Check sheet for the modelled part. Datum: model origin and axes. Units: mm. A direction names the side the tool comes from. Coordinates: 2 decimals unless noted, no trailing zeros. Order: outer loops, then holes, each group sorted by start corner. A loop starts at its lowest first (then second) coordinate and runs counter-clockwise, first axis right, second up. Notation, with made-up numbers: (85.5, 45) -> (98.5, 45) arc R20 ccw to (98.5, 52) -> close; hole circle Ø4 at (-27, 37). An arc over 180 degrees is marked (long way). Put each result on its own line as item: value. Start each with the question number.
```python
from build123d import *

# Parameters (mm, degrees)
BOSS_EXTRUDE1_DEPTH = 210
FILLET1_R           = 3
FILLET2_R           = 8
SKETCH2_R           = 3.5
SKETCH2_R_2         = 1.6
SKETCH2_W           = 10
SKETCH2_H           = 25
CUT_EXTRUDE1_DEPTH  = 111
CHAMFER1_SIZE       = 30


with BuildPart() as part:
    # Sketch1 → Boss-Extrude1 (new body)
    with BuildSketch(Plane(origin=(0, 0, 0), x_dir=(0, 0, -1), z_dir=(1, 0, 0))):
        Polygon((0, 190), (0, 0), (-110, 0), (-110, 5), (-5, 5), (-5, 190), align=None)
    extrude(amount=BOSS_EXTRUDE1_DEPTH)

    # Fillet1
    fillet1_edges = [part.edges().sort_by_distance(p)[0] for p in [
        (105, 5, 5),
    ]]
    fillet(fillet1_edges, radius=FILLET1_R)

    # Fillet2
    fillet2_edges = [part.edges().sort_by_distance(p)[0] for p in [
        (105, 0, 0),
    ]]
    fillet(fillet2_edges, radius=FILLET2_R)

    # Sketch2 → Cut-Extrude1 (cut, through all)
    with BuildSketch(Plane(origin=(0, 0, 0), x_dir=(-1, 0, 0), z_dir=(0, 0, -1))):
        with Locations((-105, 120)):
            Circle(SKETCH2_R)
        with Locations((-105, 15)):
            Circle(SKETCH2_R_2)
        with Locations((-105, 32.5)):
            Rectangle(SKETCH2_W, SKETCH2_H)
    extrude(amount=-CUT_EXTRUDE1_DEPTH, mode=Mode.SUBTRACT)

    # Chamfer1
    chamfer1_edges = [part.edges().sort_by_distance(p)[0] for p in [
        (210, 190, 2.5),
        (0, 190, 2.5),
    ]]
    chamfer(chamfer1_edges, length=CHAMFER1_SIZE)


solid = part.part
```
1) Gauge pin test, flat ends, axial feed: pin 1 (3.5 mm diameter, centred on x = 105, y = 15, fed in from +Z); pin 2 (3 mm diameter, centred on x = 93.5, z = 93.5, fed in from +Y); pin 3 (1.5 mm diameter, centred on x = 107, z = 1.5, fed in from -Y). Record the tip position at first contact, or that the pin passes through.
2) Scan lines: line 1 along Y through (x, z) = (105, 2.7); line 2 along Y through (x, z) = (105, 3.8); line 3 along Y through (x, z) = (117.5, 84.5). Record each from-to range of solid material in increasing order. Write a range as [from, to].
3) Sectioned sample at D-D (z = 54). Record the boundary of the cut face in (x, y).
4) Sectioned sample at A-A (y = 120). Record the boundary of the cut face in (x, z), plus the area to 4 significant figures.
5) Mould release check, pull along X, two halves, no side actions. Record for faces 4 (the flat face through (0, 45, 2)), 5 (the flat face through (104, 190, 3)), 6 (the flat face through (105, 20, 2)): +X half, -X half, draft (parallel to the pull), parting line (faces both ways), or undercut.
6) Sectioned sample at B-B (x = 149). Record the boundary of the cut face in (y, z), plus the area to 3 significant figures.
7) Access from +Z, -Z, +X, -X, +Y, -Y to the whole of each face (thin tool, end or side, straight path). Record for faces 1 (the flat face through (110, 32, 2)), 2 (the cylindrical face through (106.47, 2.281, 2.406)), 3 (the flat face through (104, 98, 5)).
8) Sectioned sample at C-C (x = 19). Record the boundary of the cut face in (y, z).
Entries:
1. pin 1: stops at z = 5
1. pin 2: stops at y = 5
1. pin 3: stops at y = 2.44
2. line 1: y = [2.01, 13.4], [16.6, 20], [45, 116.5], [123.5, 190]
2. line 2: y = [1.19, 13.4], [16.6, 20], [45, 116.5], [123.5, 190]
2. line 3: y = [0, 5]
3. outline: (0, 0) -> (210, 0) -> (210, 5) -> (0, 5) -> close
4. outline: (0, 0) -> (101.5, 0) -> (101.5, 5) -> (0, 5) -> close; (108.5, 0) -> (210, 0) -> (210, 5) -> (108.5, 5) -> close
4. area: 1,015 mm2
5. face 4: -X half
5. face 5: draft
5. face 6: undercut
6. outline: (0, 8) arc R8 ccw to (8, 0) -> (190, 0) -> (190, 5) -> (8, 5) arc R3 cw to (5, 8) -> (5, 110) -> (0, 110) -> close
6. area: 1,460 mm2
7. face 1: +Z, -Z
7. face 2: -Z, +X, -X, -Y
7. face 3: +Z, +X, -X, +Y
8. outline: (0, 8) arc R8 ccw to (8, 0) -> (179, 0) -> (179, 5) -> (8, 5) arc R3 cw to (5, 8) -> (5, 110) -> (0, 110) -> close
